Job drawing, mm, ordinate dimensions from the low corner. One solid piece. Give positions to 0.01 mm unless a question says otherwise; leave off trailing zeros. Order: outer loops, then holes, each group sorted by start corner. A loop starts at its lowest first (then second) coordinate and runs counter-clockwise, first axis right, second up. Notation, with made-up numbers: (-3, 75) -> (2, 75) arc R16 ccw to (2, 84) -> close; hole circle Ø11 at (72.25, 54.5). An arc over 180 degrees is marked (long way). Use CSV: the item, a comma, the result in double quotes. Start each with the question number.
1. Wall check: line 1 (X direction, y = 25, z = 4.65). Give the ranges that are in metal, low to high. Write a range as from..to.
2. Drop flat-ended pins along their axis: pin 1 (3 mm diameter, centred on x = 3.5, z = 3, fed in from +Y); pin 2 (1.8 mm diameter, centred on y = 83, z = 3.5, fed in from -X); pin 3 (8 mm diameter, centred on x = 155, y = 89, fed in from -Z); pin 4 (1.8 mm diameter, centred on y = 45.5, z = 4, fed in from +X). Give the stop position or say it passes through.
3. Cut at A-A on y = 43.5. List the corners of the cut face in (x, z).
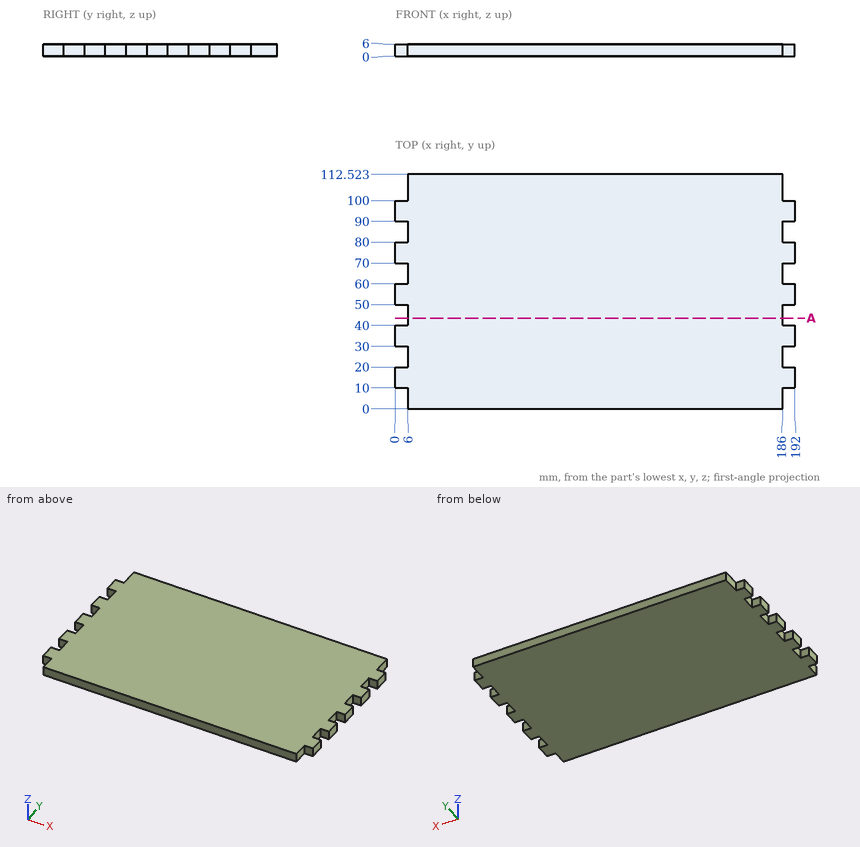
Verdict:
1,line 1,"6..186"
2,pin 1,"y = 100"
2,pin 2,"x = 6"
2,pin 3,"z = 0"
2,pin 4,"x = 186"
3,outline,"(6, 0) -> (186, 0) -> (186, 6) -> (6, 6) -> close"
